Build history of the part. All positions in model axes, mm. Round coordinates to 2 decimals unless told otherwise and drop trailing zeros. Loops run counter-clockwise (first coordinate to the right, second up) from the corner with the lowest first, then second, coordinate; pieces in that order, holes last. Notation, with made-up numbers: (75, -38.75) - (98, -38.75) arc R28 cw to (98, -9.75) - close; hole circle Ø5 at (32.25, -14). An arc over 180 degrees is marked (long way). Put each result on its own line as item: value. Start each with the question number.
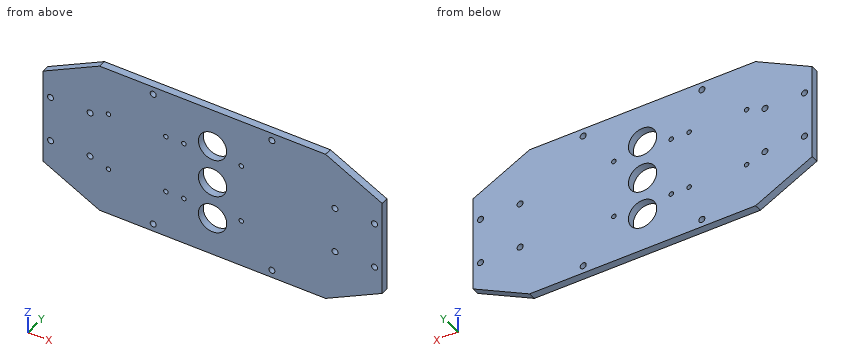
from build123d import *

# Parameters (mm, degrees)
ESQUISSE1_W             = 180
ESQUISSE1_H             = 80
BOSS_EXTRU_1_DEPTH      = 4
ENL_V_MAT_EXTRU_1_DEPTH = 4
D_GAGEMENT_M22_D        = 2.4
D_GAGEMENT_M23_D        = 2.4
D_GAGEMENT_M31_D        = 3.2
D_GAGEMENT_M31_DEPTH    = 4
ESQUISSE17_R            = 7.534005168
ESQUISSE17_R_2          = 7.5
ENL_V_MAT_EXTRU_2_DEPTH = 10


with BuildPart() as part:
    # Esquisse1 → Boss.-Extru.1 (new body)
    with BuildSketch(Plane(origin=(0, 0, 0), x_dir=(1, 0, 0), z_dir=(0, 1, 0))):
        with Locations((90, 40)):
            Rectangle(ESQUISSE1_W, ESQUISSE1_H)
    extrude(amount=BOSS_EXTRU_1_DEPTH)

    # Esquisse2 → Enlèv. mat.-Extru.1 (cut)
    with BuildSketch(Plane(origin=(0, 4, 0), x_dir=(1, 0, 0), z_dir=(0, 1, 0))):
        Polygon((0, 15), (30, 0), (0, 0), align=None)
        Polygon((30, 80), (0, 65), (0, 80), align=None)
        Polygon((150, 80), (180, 80), (180, 65), align=None)
        Polygon((180, 15), (150, 0), (180, 0), align=None)
    extrude(amount=-ENL_V_MAT_EXTRU_1_DEPTH, mode=Mode.SUBTRACT)

    # Dégagement M22 (through all)
    with Locations(Plane(origin=(0, 4, 0), x_dir=(1, 0, 0), z_dir=(0, 1, 0))):
        with Locations((74.75, 55.25), (105.25, 55.25), (105.25, 24.75), (74.75, 24.75)):
            Hole(D_GAGEMENT_M22_D / 2)

    # Dégagement M23 (through all)
    with Locations(Plane(origin=(0, 4, 0), x_dir=(1, 0, 0), z_dir=(0, 1, 0))):
        with Locations((34.75, 24.75), (65.25, 24.75), (65.25, 55.25), (34.75, 55.25)):
            Hole(D_GAGEMENT_M23_D / 2)

    # Dégagement M31
    with Locations(Plane(origin=(0, 4, 0), x_dir=(1, 0, 0), z_dir=(0, 1, 0))):
        with Locations((4, 52), (4, 28), (25, 28), (25, 52), (58.5, 76), (58.5, 4), (121.5, 4), (121.5, 76), (155, 52), (176, 52), (176, 28), (155, 28)):
            Hole(D_GAGEMENT_M31_D / 2, depth=D_GAGEMENT_M31_DEPTH)

    # Esquisse17 → Enlèv. mat.-Extru.2 (cut)
    with BuildSketch(Plane(origin=(0, 4, 0), x_dir=(1, 0, 0), z_dir=(0, 1, 0))):
        with Locations((90, 60)):
            Circle(ESQUISSE17_R)
        with Locations((90, 40)):
            Circle(ESQUISSE17_R_2)
        with Locations((90, 20)):
            Circle(ESQUISSE17_R_2)
    extrude(amount=-ENL_V_MAT_EXTRU_2_DEPTH, mode=Mode.SUBTRACT)


solid = part.part
Item 1: Drill centre lines: probe 1 along X at (y, z) = (2.75, -52); probe 2 along Z at (x, y) = (105.25, 2.55); probe 3 along Z at (x, y) = (58.5, 1.85). Where is each one in solid material? Low to high. Write a range as [from, to].
Item 2: Slice it at C-C (z = -60). Give the cut face in (x, y).
Item 3: Slice it at A-A (z = -76). Give the cut face in (x, y), plus the area to 3 significant figures.
Item 4: Drop flat-ended pins along their axis: pin 1 Ø1.9 at (x, z) = (155, -28) entering from -Y; pin 2 Ø3.5 at (x, z) = (25, -28) entering from +Y. Give the stop position or say it passes through.
Item 5: Slice it at B-B (x = 4). Give the cut face in (y, z).
Item 6: Slice it at D-D (x = 90). Give the cut face in (y, z).
Computed values:
1. probe 1: x = [0, 2.4], [5.6, 23.4], [26.6, 153.4], [156.6, 174.4], [177.6, 180]
1. probe 2: z = [-80, -56.45], [-54.05, -25.95], [-23.55, 0]
1. probe 3: z = [-80, -77.6], [-74.4, -5.6], [-2.4, 0]
2. outline: (0, 0) - (82.47, 0) - (82.47, 4) - (0, 4) - close; (97.53, 0) - (180, 0) - (180, 4) - (97.53, 4) - close
3. outline: (22, 0) - (56.9, 0) - (56.9, 4) - (22, 4) - close; (60.1, 0) - (119.9, 0) - (119.9, 4) - (60.1, 4) - close; (123.1, 0) - (158, 0) - (158, 4) - (123.1, 4) - close
3. area: 518 mm^2
4. pin 1: passes through
4. pin 2: stops at y = 4
5. outline: (0, -67) - (4, -67) - (4, -53.6) - (0, -53.6) - close; (0, -50.4) - (4, -50.4) - (4, -29.6) - (0, -29.6) - close; (0, -26.4) - (4, -26.4) - (4, -13) - (0, -13) - close
6. outline: (0, -80) - (4, -80) - (4, -67.53) - (0, -67.53) - close; (0, -52.47) - (4, -52.47) - (4, -47.5) - (0, -47.5) - close; (0, -32.5) - (4, -32.5) - (4, -27.5) - (0, -27.5) - close; (0, -12.5) - (4, -12.5) - (4, 0) - (0, 0) - close
